For this review, use the dimensioned drawing (mm, ordinates from the lowest corner) and the shaded views. Give positions to 0.01 mm unless a question says otherwise; leave off trailing zeros. Order: outer loops, then holes, each group sorted by start corner. A loop starts at its lowest first (then second) coordinate and runs counter-clockwise, first axis right, second up.
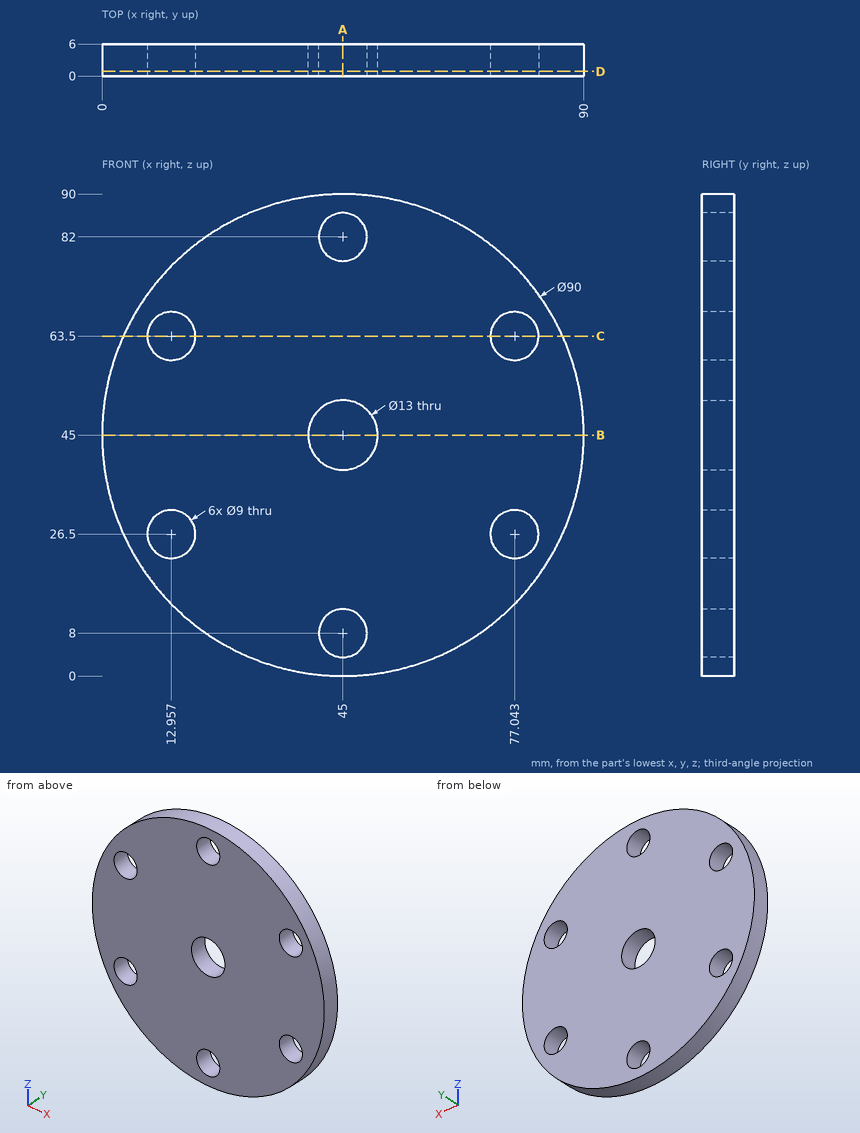
1. Take a section at C-C (z = 63.5). State the section outline as (x, y) points.
Recorded:
outline: (3.98, 0) - (8.46, 0) - (8.46, 6) - (3.98, 6) - close; (17.46, 0) - (72.54, 0) - (72.54, 6) - (17.46, 6) - close; (81.54, 0) - (86.02, 0) - (86.02, 6) - (81.54, 6) - close
2. For line 1 along Z through (x, y) = (45, 3.3); line 2 along Z through (x, y) = (39.5, 4.4); line 3 along X through (y, z) = (5.6, 32), list the stretches that pass through material, from the lowest coordinate up.
Recorded:
line 1: z = 0 to 3.5, 12.5 to 38.5, 51.5 to 77.5, 86.5 to 90
line 2: z = 0.34 to 41.54, 48.46 to 89.66
line 3: x = 1.92 to 88.08
3. For pin 1 (2 mm diameter, centred on y = 2.5, z = 54, fed in from +X); pin 2 (1.5 mm diameter, centred on x = 9, y = 1, fed in from -Z), all flat-tipped, find the tip position at first contact; note any pin that passes through.
Recorded:
pin 1: stops at x = 89.28
pin 2: stops at z = 17.03
4. Take a section at B-B (z = 45). State the section outline as (x, y) points, then the cut area to 3 significant figures.
Recorded:
outline: (0, 0) - (38.5, 0) - (38.5, 6) - (0, 6) - close; (51.5, 0) - (90, 0) - (90, 6) - (51.5, 6) - close
area: 462 mm2
5. Take a section at A-A (x = 45). State the section outline as (y, z) points.
Recorded:
outline: (0, 0) - (6, 0) - (6, 3.5) - (0, 3.5) - close; (0, 12.5) - (6, 12.5) - (6, 38.5) - (0, 38.5) - close; (0, 51.5) - (6, 51.5) - (6, 77.5) - (0, 77.5) - close; (0, 86.5) - (6, 86.5) - (6, 90) - (0, 90) - close
6. Take a section at D-D (y = 0.9). State the section outline as (x, z) points.
Recorded:
outline: circle Ø90 at (45, 45); hole circle Ø9 at (12.96, 26.5); hole circle Ø9 at (12.96, 63.5); hole circle Ø13 at (45, 45); hole circle Ø9 at (45, 8); hole circle Ø9 at (45, 82); hole circle Ø9 at (77.04, 26.5); hole circle Ø9 at (77.04, 63.5)
